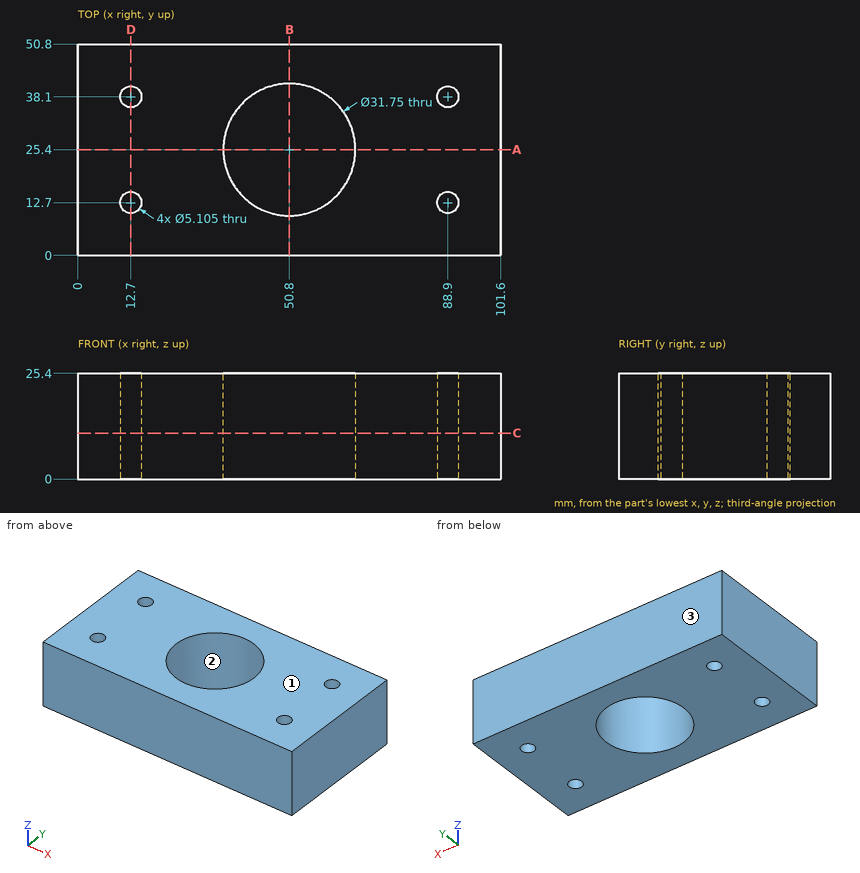
Print and shaded views of the part. All mm, measured from the part's lowest x, y and z. Coordinates: 2 decimals unless noted, no trailing zeros. Order: outer loops, then holes, each group sorted by start corner. A loop starts at its lowest first (then second) coordinate and runs counter-clockwise, first axis right, second up. Notation, with made-up numbers: (-6.75, 83) - (31.25, 83) arc R27 cw to (31.25, 122) - close; hole circle Ø8 at (-18, 42.5). An arc over 180 degrees is marked (long way). Return JSON: item names as keys, results as strings. Group by question number.
Item 1: Cut at D-D (x = 12.7). List the corners of the cut face in (y, z).
Item 2: Cut at A-A (y = 25.4). List the corners of the cut face in (x, z) (1 decimal), plus the area to 3 significant figures.
Item 3: Cut at C-C (z = 11). State how many separate pieces and enclosed holes the cut face has, plus the area to 3 significant figures.
Item 4: Pull direction Y, two halves, no side cores. Call the marked faces 1, 2 and 3: pulls with the +Y half, pulls with the -Y half, needs draft (parallel to the pull), parting line crosses it, or undercut.
Item 5: Cut at B-B (x = 50.8). List the corners of the cut face in (y, z) (1 decimal), plus the area to 3 significant figures.
Item 6: Drill centre lines: probe 1 along Y at (x, z) = (88.9, 9.25); probe 2 along Y at (x, z) = (63, 7.5) (1 decimal); probe 3 along Y at (x, z) = (50.8, 12) (1 decimal). Where is each one in solid material? Low to high. Write a range as from..to.
Check values:
{
 "1": {"outline": "(0, 0) - (10.15, 0) - (10.15, 25.4) - (0, 25.4) - close; (15.25, 0) - (35.55, 0) - (35.55, 25.4) - (15.25, 25.4) - close; (40.65, 0) - (50.8, 0) - (50.8, 25.4) - (40.65, 25.4) - close"},
 "2": {"outline": "(0, 0) - (34.9, 0) - (34.9, 25.4) - (0, 25.4) - close; (66.7, 0) - (101.6, 0) - (101.6, 25.4) - (66.7, 25.4) - close", "area": "1,770 mm2"},
 "3": {"separate pieces": "1", "enclosed holes": "5", "area": "4,290 mm2"},
 "4": {"face 1": "needs draft", "face 2": "undercut", "face 3": "pulls with the +Y half"},
 "5": {"outline": "(0, 0) - (9.5, 0) - (9.5, 25.4) - (0, 25.4) - close; (41.3, 0) - (50.8, 0) - (50.8, 25.4) - (41.3, 25.4) - close", "area": "484 mm2"},
 "6": {"probe 1": "y = 0..10.15, 15.25..35.55, 40.65..50.8", "probe 2": "y = 0..15.2, 35.6..50.8", "probe 3": "y = 0..9.5, 41.3..50.8"}
}
